from build123d import *

# Parameters (mm, degrees)
BOSS_EXTRUDE1_DEPTH = 1
SKETCH2_R           = 2.5
CUT_EXTRUDE1_DEPTH  = 20
SKETCH3_W           = 5
SKETCH3_H           = 5
CUT_EXTRUDE2_DEPTH  = 10
SKETCH4_R           = 3.881431072
CUT_EXTRUDE3_DEPTH  = 10


with BuildPart() as part:
    # Sketch1 → Boss-Extrude1 (new body)
    with BuildSketch(Plane(origin=(0, 0, 0), x_dir=(1, 0, 0), z_dir=(0, 1, 0))):
        with BuildLine():
            Line((-19.801702617, 0), (17.198297383, 0))
            Line((17.198297383, 0), (17.198297383, 37))
            ThreePointArc((17.198297383, 37), (30.611248287, 20.881727984), (28.698297383, 0))
            Line((28.698297383, 0), (28.698297383, -45))
            Line((28.698297383, -45), (-31.301702617, -45))
            Line((-31.301702617, -45), (-31.301702617, 0))
            ThreePointArc((-31.301702617, 0), (-33.214653521, 20.881727984), (-19.801702617, 37))
            Line((-19.801702617, 37), (-19.801702617, 0))
        make_face()
    extrude(amount=BOSS_EXTRUDE1_DEPTH)

    # Sketch2 → Cut-Extrude1 (cut)
    with BuildSketch(Plane(origin=(0, 1, 0), x_dir=(1, 0, 0), z_dir=(0, 1, 0))):
        with Locations(Location((-1.301702617, -25, 0), (0, 0, 270))):
            Circle(SKETCH2_R)
    extrude(amount=-CUT_EXTRUDE1_DEPTH, mode=Mode.SUBTRACT)

    # Sketch3 → Cut-Extrude2 (cut)
    with BuildSketch(Plane.XZ):
        with Locations((13.198297383, 9.5)):
            Rectangle(SKETCH3_W, SKETCH3_H)
        with Locations((-15.801702617, 9.5)):
            Rectangle(SKETCH3_W, SKETCH3_H)
    extrude(amount=-CUT_EXTRUDE2_DEPTH, mode=Mode.SUBTRACT)

    # Sketch4 → Cut-Extrude3 (cut)
    with BuildSketch(Plane.XZ):
        with Locations(Location((13.198297383, 9.5, 0), (0, 0, 270))):
            Circle(SKETCH4_R)
        with Locations(Location((-15.801702617, 9.5, 0), (0, 0, 90))):
            Circle(SKETCH4_R)
    extrude(amount=-CUT_EXTRUDE3_DEPTH, mode=Mode.SUBTRACT)


solid = part.part
Design review of the part built by this model. Coordinates are the model's own, in mm. Coordinates: 2 decimals unless noted, no trailing zeros. Write each loop counter-clockwise with the first axis right and the second up, starting at its lowest first coordinate (ties: lowest second). Pieces come first, ordered by that corner, then holes. Notation, with made-up numbers: (39, -20.75) - (67, -20.75) arc R24 cw to (67, 9.25) - close; hole circle Ø3 at (-8.75, 41.25). An arc over 180 degrees is marked (long way). Use one line per item in the form item = value.
Q1. Insertion check: pin 1 Ø7 at (x, z) = (-15.8, 9.5) entering from +Y. The pin has a flat end and moves straight along its axis. Give the tip position at first contact, or say it passes through.
Taken from the geometry:
pin_1 = through
Q2. For probe 1 along X at (y, z) = (0.3, 9.5); probe 2 along Z at (x, y) = (13.5, 0.2); probe 3 along X at (y, z) = (0.8, 40), list the stretches that pass through material, from the lowest coordinate up.
Taken from the geometry:
probe_1 = -31.3 to -19.68, -11.92 to 9.32, 17.08 to 28.7
probe_2 = 0 to 5.63, 13.37 to 45
probe_3 = -31.3 to 28.7
Q3. Consider section A-A (z = 9.5). Write out the cut boundary in (x, y), plus the area to 3 significant figures.
Taken from the geometry:
outline = (-31.3, 0) - (-19.68, 0) - (-19.68, 1) - (-31.3, 1) - close; (-11.92, 0) - (9.32, 0) - (9.32, 1) - (-11.92, 1) - close; (17.08, 0) - (28.7, 0) - (28.7, 1) - (17.08, 1) - close
area = 44.5 mm^2
Q4. The part is to be moulded in two halves that separate along X. For faces 1 (the cylindrical face through (-1.192, 0.507, 22.502)), 2 (the flat face through (-1, 1, 13)), 3 (the cylindrical face through (-19.65, 0.49, 8.99)), 4 (the cylindrical face through (30.52, 0.49, -21.17)), say which applies: +X half, -X half, draft (parallel to the pull), parting line (faces both ways), or undercut.
Taken from the geometry:
face_1 = undercut
face_2 = draft
face_3 = undercut
face_4 = +X half
Q5. Consider section D-D (y = 0.75). Write out the cut boundary in (x, z), plus the area to 3 significant figures.
Taken from the geometry:
outline = (-31.3, 0) arc R27.4 ccw to (-19.8, -37) - (-19.8, 0) - (17.2, 0) - (17.2, -37) arc R27.4 ccw to (28.7, 0) - (28.7, 45) - (-31.3, 45) - close; hole circle Ø7.76 at (-15.8, 9.5); hole circle Ø5 at (-1.3, 25); hole circle Ø7.76 at (13.2, 9.5)
area = 3,440 mm^2
Q6. Consider section B-B (z = 25). Write out the cut boundary in (x, y).
Taken from the geometry:
outline = (-31.3, 0) - (-3.8, 0) - (-3.8, 1) - (-31.3, 1) - close; (1.2, 0) - (28.7, 0) - (28.7, 1) - (1.2, 1) - close
Q7. Consider section C-C (x = -18). Write out the cut boundary in (y, z), plus the area to 3 significant figures.
Taken from the geometry:
outline = (0, 0) - (1, 0) - (1, 6.3) - (0, 6.3) - close; (0, 12.7) - (1, 12.7) - (1, 45) - (0, 45) - close
area = 38.6 mm^2
